Work out the finished part from the listing and answer in its coordinate system (mm). Face numbers are marked on the shaded views. Give positions to 0.01 mm unless a question says otherwise; leave off trailing zeros. Loops run counter-clockwise (first coordinate to the right, second up) from the corner with the lowest first, then second, coordinate; pieces in that order, holes last. Notation, with made-up numbers: M -18.5,78 L 34.5,78 A11 ccw 34.5,93 Z; hole C -34.5,56 d6. An arc over 180 degrees is marked long. Use a Markdown table: item, result.
```python
from build123d import *

# Parameters (mm, degrees)
SKETCH1_R           = 25
SKETCH1_R_2         = 10
BOSS_EXTRUDE1_DEPTH = 12
CUT_EXTRUDE1_DEPTH  = 38.336309405


with BuildPart() as part:
    # Sketch1 → Boss-Extrude1 (new body)
    with BuildSketch(Plane(origin=(0, 0, 0), x_dir=(0, 0, -1), z_dir=(1, 0, 0))):
        Circle(SKETCH1_R)
        Circle(SKETCH1_R_2, mode=Mode.SUBTRACT)
    extrude(amount=BOSS_EXTRUDE1_DEPTH)

    # Sketch2 → Cut-Extrude1 (cut, through all)
    with BuildSketch(Plane(origin=(12, 0, 0), x_dir=(0, 0, -1), z_dir=(1, 0, 0))):
        with BuildLine():
            ThreePointArc((-2, 9.797958971), (-1.00508962, 9.94936153), (0, 10))
            Line((0, 10), (0, 10.797958971))
            Line((0, 10.797958971), (-2, 10.797958971))
            Line((-2, 10.797958971), (-2, 9.797958971))
        make_face()
        with BuildLine():
            Line((0, 10.797958971), (0, 10))
            ThreePointArc((0, 10), (1.00508962, 9.94936153), (2, 9.797958971))
            Line((2, 9.797958971), (2, 10.797958971))
            Line((2, 10.797958971), (0, 10.797958971))
        make_face()
    extrude(amount=-CUT_EXTRUDE1_DEPTH, mode=Mode.SUBTRACT)


solid = part.part
```
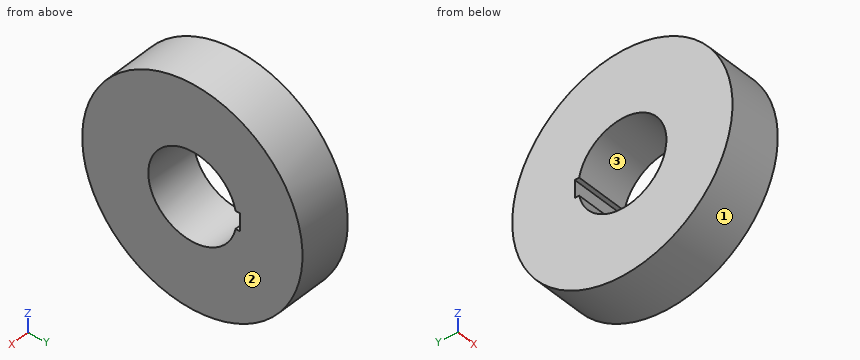
(1) A cutting plane is placed at C-C (x = 5.75). Write down the section's boundary in (y, z), and give its area (3 significant figures).
Entries:
| item | result |
|---|---|
| outline | C 0,0 d50; hole M 9.8,-2 L 10.8,-2 L 10.8,2 L 9.8,2 A10 ccw long Z |
| area | 1,650 mm² |
(2) Consider probe 1 along Y at (x, z) = (4.5, 0); probe 2 along Y at (x, z) = (9.25, 7). Determine where each line is inside the solid, lowest interval first. Write a range as [from, to].
Entries:
| item | result |
|---|---|
| probe 1 | y = [-25, -10], [10.8, 25] |
| probe 2 | y = [-24, -7.14], [7.14, 24] |
(3) The mould has two halves that part along Y. Classify the marked faces 1, 2 and 3: released by +Y, released by -Y, zero draft, split by the parting line, or undercut.
Entries:
| item | result |
|---|---|
| face 1 | split by the parting line |
| face 2 | zero draft |
| face 3 | undercut |
(4) Given P1, Ø4, axis at x = 6, y = -15.5, coming from the +Z side; P2, Ø1.5, axis at x = 8, z = -7, coming from the -Y side; P3, Ø3, axis at x = 6.5, z = 0.5, coming from the -Y side, each flat-ended and moving along its own axis, determine where each tip first touches the part or whether it passes through.
Entries:
| item | result |
|---|---|
| P1 | stops at z = 21.04 |
| P2 | stops at y = -24.21 |
| P3 | stops at y = -25 |
(5) A cutting plane is placed at D-D (z = 15). Write down the section's boundary in (x, y).
Entries:
| item | result |
|---|---|
| outline | M 0,-20 L 12,-20 L 12,20 L 0,20 Z |
(6) A cutting plane is placed at B-B (z = 0). Write down the section's boundary in (x, y), and give its area (3 significant figures).
Entries:
| item | result |
|---|---|
| outline | M 0,-25 L 12,-25 L 12,-10 L 0,-10 Z; M 0,10.8 L 12,10.8 L 12,25 L 0,25 Z |
| area | 350 mm² |
(7) A cutting plane is placed at A-A (y = 0). Write down the section's boundary in (x, z), and give its area (3 significant figures).
Entries:
| item | result |
|---|---|
| outline | M 0,-25 L 12,-25 L 12,-10 L 0,-10 Z; M 0,10 L 12,10 L 12,25 L 0,25 Z |
| area | 360 mm² |
